from build123d import *

# Parameters (mm, degrees)
SKETCH1_R           = 4.7625
BOSS_EXTRUDE1_DEPTH = 3.96875
FILLET1_R           = 10
FILLET2_R           = 15


with BuildPart() as part:
    # Sketch1 → Boss-Extrude1 (new body)
    with BuildSketch(Plane(origin=(0, 0, 0), x_dir=(1, 0, 0), z_dir=(0, 1, 0))):
        with BuildLine():
            Line((-68.7, 0), (-68.7, 19.3))
            Line((-68.7, 19.3), (-34.35, 62.254365319))
            Line((-34.35, 62.254365319), (0, 19.3))
            Line((0, 19.3), (0, 0))
            ThreePointArc((0, 0), (-34.35, -3.905912777), (-68.7, 0))
        make_face()
        with Locations((-34.35, 37)):
            Circle(SKETCH1_R, mode=Mode.SUBTRACT)
        with BuildLine():
            Line((-58.35, 12), (-10.35, 12))
            ThreePointArc((-10.35, 12), (-7.35, 9), (-10.35, 6))
            Line((-10.35, 6), (-58.35, 6))
            ThreePointArc((-58.35, 6), (-61.35, 9), (-58.35, 12))
        make_face(mode=Mode.SUBTRACT)
    extrude(amount=BOSS_EXTRUDE1_DEPTH)

    # Fillet1
    fillet1_edges = [part.edges().sort_by_distance(p)[0] for p in [
        (-68.7, 1.984375, 0),
        (-68.7, 1.984375, -19.3),
        (0, 1.984375, -19.3),
        (0, 1.984375, 0),
    ]]
    fillet(fillet1_edges, radius=FILLET1_R)

    # Fillet2
    fillet2_edges = [part.edges().sort_by_distance(p)[0] for p in [
        (-34.35, 1.984375, -62.254365319),
    ]]
    fillet(fillet2_edges, radius=FILLET2_R)


solid = part.part
Input: part model. Units: mm. Frame: model coordinates. A direction names the side the tool comes from. Round coordinates to 2 decimals unless told otherwise and drop trailing zeros. Order: outer loops, then holes, each group sorted by start corner. A loop starts at its lowest first (then second) coordinate and runs counter-clockwise, first axis right, second up. Notation, with made-up numbers: (52, 32.5) - (109, 32.5) arc R29 cw to (109, 59.5) - close; hole circle Ø2 at (-31, 3.25). An arc over 180 degrees is marked (long way). Use a Markdown table: item, result.
1. Mould query, pull axis Z, two halves, no side actions, for faces 3 (the face through (-34, 0, -25)), 4 (the face through (-33.983, 1.957, 3.905)), 5 (the face through (-7.35, 1.96, -9.07)), 6 (the face through (-61.35, 1.96, -8.93)). Classes: +Z half, -Z half, draft (parallel to the pull), parting line (faces both ways), or undercut.
Evaluation:
| item | result |
|---|---|
| face 3 | draft |
| face 4 | +Z half |
| face 5 | undercut |
| face 6 | undercut |
2. Access query for faces 1 (the face through (-34, 2, -6)), 2 (the face through (-56.43, 1.957, -34.643)). Directions: +Z, -Z, +X, -X, +Y, -Y. A direction counts if a zero-diameter tool reaches every point of the face in a straight line with its end or side. Return the directions, or none.
Evaluation:
| item | result |
|---|---|
| face 1 | +Y, -Y |
| face 2 | -Z, -X, +Y, -Y |
3. Section D-D on x = -44. Return the cut outline in (y, z).
Evaluation:
| item | result |
|---|---|
| outline | (0, -49.72) - (3.97, -49.72) - (3.97, -12) - (0, -12) - close; (0, -6) - (3.97, -6) - (3.97, 3.6) - (0, 3.6) - close |
4. First-contact query: pin 1 (1.5 mm diameter, centred on y = 2, z = -31.5, fed in from +X); pin 2 (1.2 mm diameter, centred on x = -39, y = 1.5, fed in from +Z); pin 3 (1 mm diameter, centred on y = 2, z = -19, fed in from -X). Flat tips, straight axial feed; report the tip coordinate or a pass-through.
Evaluation:
| item | result |
|---|---|
| pin 1 | x = -9.16 |
| pin 2 | z = 3.85 |
| pin 3 | x = -68.33 |
5. Section C-C on y = 0.6. State how many separate pieces and enclosed holes the cut face has, then the cut area to 3 significant figures.
Evaluation:
| item | result |
|---|---|
| separate pieces | 1 |
| enclosed holes | 2 |
| area | 2,480 mm^2 |
6. Section B-B on z = -9. Return the cut outline in (x, y), then the cut area to 3 significant figures.
Evaluation:
| item | result |
|---|---|
| outline | (-68.7, 0) - (-61.35, 0) - (-61.35, 3.97) - (-68.7, 3.97) - close; (-7.35, 0) - (0, 0) - (0, 3.97) - (-7.35, 3.97) - close |
| area | 58.3 mm^2 |
7. Section A-A on x = -34.35. Return the cut outline in (y, z), then the cut area to 3 significant figures.
Evaluation:
| item | result |
|---|---|
| outline | (0, -53.24) - (3.97, -53.24) - (3.97, -41.76) - (0, -41.76) - close; (0, -32.24) - (3.97, -32.24) - (3.97, -12) - (0, -12) - close; (0, -6) - (3.97, -6) - (3.97, 3.91) - (0, 3.91) - close |
| area | 165 mm^2 |
8. Material intervals for probe 1 along X at (y, z) = (2.8, -37); probe 2 along Z at (x, y) = (-27, 1.95); probe 3 along Z at (x, y) = (-48, 2.05), sorted ascending.
Evaluation:
| item | result |
|---|---|
| probe 1 | -54.55 to -39.11, -29.59 to -14.15 |
| probe 2 | -51.31 to -12, -6 to 3.73 |
| probe 3 | -45.19 to -12, -6 to 3.3 |
